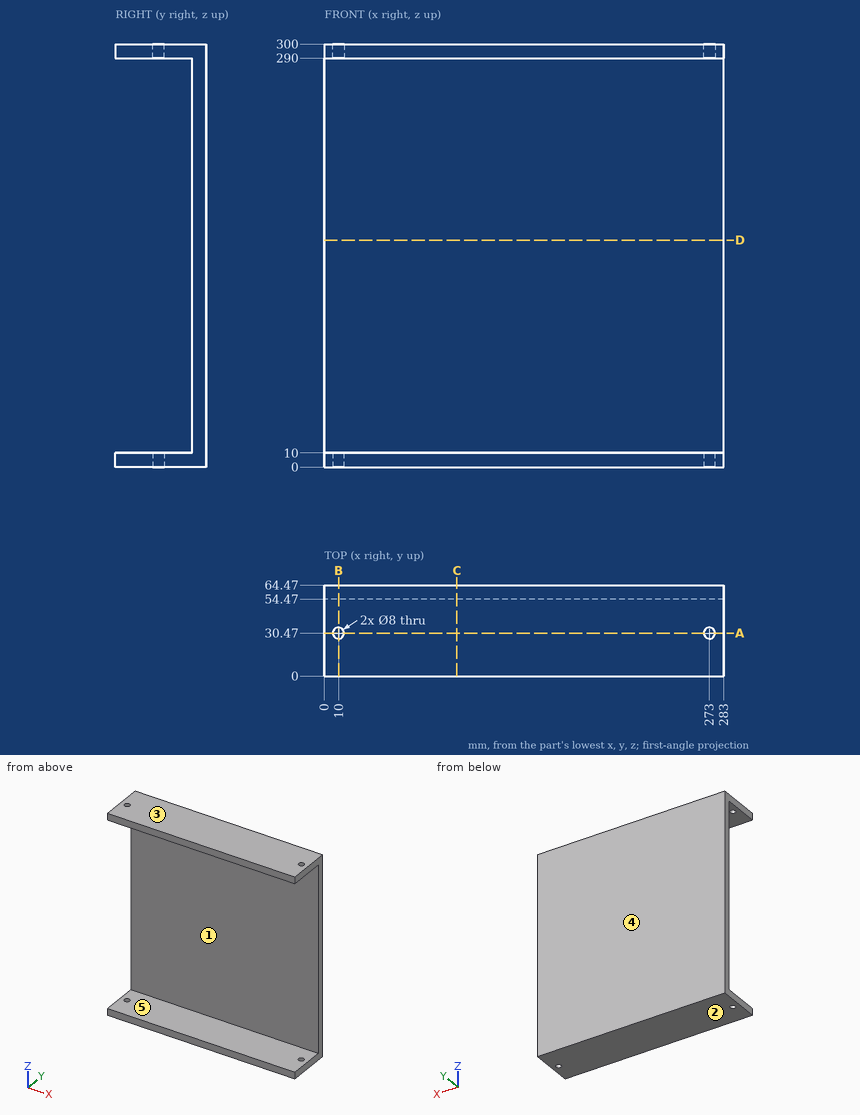
Design review of the part shown in the three views and the two pictorial views. Dimensions are in mm from the part's minimum x, y and z. A direction names the side the tool comes from. Coordinates: 2 decimals unless noted, no trailing zeros. Loops run counter-clockwise (first coordinate to the right, second up) from the corner with the lowest first, then second, coordinate; pieces in that order, holes last. Notation, with made-up numbers: M 3.25,26.25 L 17.25,26.25 A21 cw 17.25,43.25 Z; hole C 49.25,-12.5 d5. An arc over 180 degrees is marked long. Put each result on its own line as item: value. Start each with the question number.
Q1. Add section C-C (x = 94). Write out the cut boundary in (y, z).
Q2. The part is to be moulded in two halves that separate along Z. For the marked faces 3, 4 and 5, say which applies: +Z half, -Z half, draft (parallel to the pull), parting line (faces both ways), or undercut.
Q3. Add section A-A (y = 30.47). Write out the cut boundary in (x, z).
Q4. For the marked faces 1 and 2, list the 3-axis set-ups (+Z, -Z, +X, -X, +Y, -Y) from which the entire face can be reached by the end or side of a thin tool; tool diameter is ignored.
Q5. Add section D-D (z = 161). Write out the cut boundary in (x, y), and give its area (3 significant figures).
Q6. Clearance check with flat-ended pins moving along their axes: pin 1 (4 mm diameter, centred on x = 111.5, z = 62, fed in from -Y); pin 2 (6.5 mm diameter, centred on x = 273, y = 30.47, fed in from -Z). State where each tip first meets the part, or that it passes through.
Q7. Add section B-B (x = 10). Write out the cut boundary in (y, z).
Q8. Wall thickness on line 1 (Z direction, x = 138, y = 45); line 2 (Y direction, x = 10, z = 296); line 3 (Y direction, x = 202, z = 154.5): over which ranges is each line inside the solid? List them lowest first.
Answers:
1. outline: M 0,0 L 64.47,0 L 64.47,300 L 0,300 L 0,290 L 54.47,290 L 54.47,10 L 0,10 Z
2. face 3: +Z half
2. face 4: draft
2. face 5: undercut
3. outline: M 0,0 L 6,0 L 6,10 L 0,10 Z; M 0,290 L 6,290 L 6,300 L 0,300 Z; M 14,0 L 269,0 L 269,10 L 14,10 Z; M 14,290 L 269,290 L 269,300 L 14,300 Z; M 277,0 L 283,0 L 283,10 L 277,10 Z; M 277,290 L 283,290 L 283,300 L 277,300 Z
4. face 1: +X, -X, -Y
4. face 2: -Z, +X, -X, +Y, -Y
5. outline: M 0,54.47 L 283,54.47 L 283,64.47 L 0,64.47 Z
5. area: 2,830 mm^2
6. pin 1: stops at y = 54.47
6. pin 2: passes through
7. outline: M 0,0 L 26.47,0 L 26.47,10 L 0,10 Z; M 0,290 L 26.47,290 L 26.47,300 L 0,300 Z; M 34.47,0 L 64.47,0 L 64.47,300 L 34.47,300 L 34.47,290 L 54.47,290 L 54.47,10 L 34.47,10 Z
8. line 1: z = 0 to 10, 290 to 300
8. line 2: y = 0 to 26.47, 34.47 to 64.47
8. line 3: y = 54.47 to 64.47
